from build123d import *

# Parameters (mm, degrees)
SKETCH_1_W          = 8
SKETCH_1_H          = 8
EXTRUDE_1_DEPTH     = 22
SKETCH_2_R          = 1.5
CUT_EXTRUDE_1_DEPTH = 9
SKETCH_3_R          = 1.5
CUT_EXTRUDE_2_DEPTH = 9


with BuildPart() as part:
    # 草图1 → 凸台-拉伸1 (new body)
    with BuildSketch(Plane.XY):
        Rectangle(SKETCH_1_W, SKETCH_1_H)
    extrude(amount=EXTRUDE_1_DEPTH)

    # 草图2 → 切除-拉伸1 (cut, through all)
    with BuildSketch(Plane(origin=(0, 4, 0), x_dir=(1, 0, 0), z_dir=(0, 1, 0))):
        with Locations((0, -5)):
            Circle(SKETCH_2_R)
        with Locations((0, -13)):
            Circle(SKETCH_2_R)
    extrude(amount=-CUT_EXTRUDE_1_DEPTH, mode=Mode.SUBTRACT)

    # 草图3 → 切除-拉伸2 (cut, through all)
    with BuildSketch(Plane(origin=(4, 0, 0), x_dir=(0, 0, -1), z_dir=(1, 0, 0))):
        with Locations((-17, 0)):
            Circle(SKETCH_3_R)
        with Locations((-9, 0)):
            Circle(SKETCH_3_R)
    extrude(amount=-CUT_EXTRUDE_2_DEPTH, mode=Mode.SUBTRACT)


solid = part.part
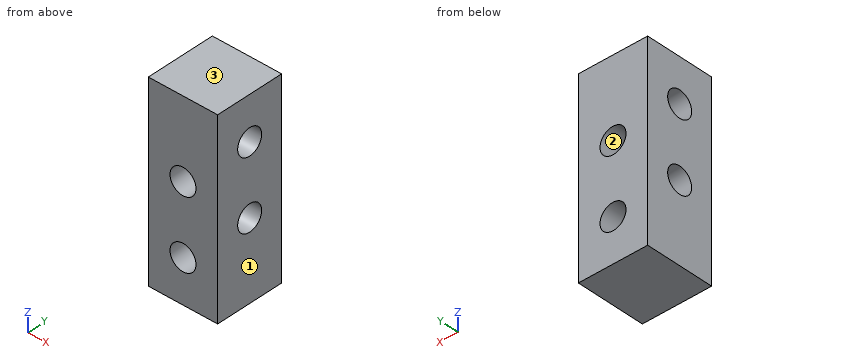
Work out the finished part from the listing and answer in its coordinate system (mm). Face numbers are marked on the shaded views. Coordinates: 2 decimals unless noted, no trailing zeros. Write each loop counter-clockwise with the first axis right and the second up, starting at its lowest first coordinate (ties: lowest second). Pieces come first, ordered by that corner, then holes.
1. Consider line 1 along Y through (x, z) = (1.25, 17); line 2 along Z through (x, y) = (0, -0.75). Determine where each line is inside the solid, lowest interval first.
Results list:
line 1: y = -4 to -1.5, 1.5 to 4
line 2: z = 0 to 3.5, 6.5 to 7.7, 10.3 to 11.5, 14.5 to 15.7, 18.3 to 22
2. The part is cut by section C-C, the plane y = -0.5. Write down the section's boundary in (x, z), and give its area (3 significant figures).
Results list:
outline: (-4, 0) - (4, 0) - (4, 7.59) - (-4, 7.59) - close; (-4, 10.41) - (4, 10.41) - (4, 15.59) - (-4, 15.59) - close; (-4, 18.41) - (4, 18.41) - (4, 22) - (-4, 22) - close; hole circle Ø3 at (0, 5); hole circle Ø3 at (0, 13)
area: 117 mm2
3. Flat-ended cylindrical pins translate along their axes: pin 1 (2.5 mm diameter, centred on y = 0, z = 17, fed in from -X); pin 2 (4 mm diameter, centred on x = -2.5, y = -1.5, fed in from -Z). Find the tip coordinate at first contact, or state that the pin passes through.
Results list:
pin 1: passes through
pin 2: stops at z = 0
4. For a pull along X with two mould halves and no side action, classify the marked faces 1, 2 and 3 as +X half, -X half, draft (parallel to the pull), parting line (faces both ways), or undercut.
Results list:
face 1: +X half
face 2: undercut
face 3: draft
5. The part is cut by section A-A, the plane x = 0. Write down the section's boundary in (y, z).
Results list:
outline: (-4, 0) - (4, 0) - (4, 3.5) - (-4, 3.5) - close; (-4, 6.5) - (4, 6.5) - (4, 11.5) - (-4, 11.5) - close; (-4, 14.5) - (4, 14.5) - (4, 22) - (-4, 22) - close; hole circle Ø3 at (0, 9); hole circle Ø3 at (0, 17)
6. The part is cut by section D-D, the plane x = 3. Write down the section's boundary in (y, z), and give its area (3 significant figures).
Results list:
outline: (-4, 0) - (4, 0) - (4, 22) - (-4, 22) - close; hole circle Ø3 at (0, 9); hole circle Ø3 at (0, 17)
area: 162 mm2
7. The part is cut by section B-B, the plane z = 5. Write down the section's boundary in (x, y), and give its area (3 significant figures).
Results list:
outline: (-4, -4) - (-1.5, -4) - (-1.5, 4) - (-4, 4) - close; (1.5, -4) - (4, -4) - (4, 4) - (1.5, 4) - close
area: 40.0 mm2
